Autodesk Inventor part; units mm, degrees
ref_plane "YZ Plane" through (0, 0, 0) normal (1, 0, 0) x (0, 1, 0)
ref_plane "XZ Plane" through (0, 0, 0) normal (0, 1, 0) x (-1, 0, 0)
ref_plane "XY Plane" through (0, 0, 0) normal (0, 0, 1) x (1, 0, 0)
sketch "Sketch1" plane through (0, 0, 0) normal (0, 0, 1) x (1, 0, 0)
  line L0 (0, 0) -> (31.75, 0) construction
  line L1 (31.75, 0) -> (44.45, 0)
  line L2 (44.45, 0) -> (44.45, -19.05)
  line L3 (44.45, -19.05) -> (38.1, -30.0485)
  line L4 (38.1, -30.0485) -> (38.1, -42.7485)
  line L5 (38.1, -42.7485) -> (44.45, -53.747)
  line L6 (44.45, -53.747) -> (44.45, -88.9)
  line L7 (44.45, -88.9) -> (31.75, -88.9)
  line L8 (31.75, -88.9) -> (31.75, 0)
  line L9 (0, 0) -> (0, -152.4)
  dimension "d0" = 31.75
  dimension "d1" = 12.7
  dimension "d2" = 6.35
  dimension "d3" = 150
  dimension "d4" = 19.05
  dimension "d5" = 88.9
  dimension "d6" = 150
  dimension "d7" = 12.7
  dimension "d9" = 152.4
revolve "Revolution1" add sketch "Sketch1" angle 270 about axis through (0, 0, 0) along (0, -1, 0)
fillet "Fillet1" radius 12.7 2 edges at (-31.4309, -19.05, 31.4309) (-31.4309, -53.747, 31.4309)
fillet "Fillet1" radius 6.35 2 edges at (-26.9408, -42.7485, 26.9408) (-26.9408, -30.0485, 26.9408)
equation "\"d6\" = d3"
properties part number "Foam Weight Shifter Pad 1"
Verification items for the finished model (mm, model axes). A direction names the side the tool comes from. Give positions to 0.01 mm unless a question says otherwise; leave off trailing zeros. Order: outer loops, then holes, each group sorted by start corner. A loop starts at its lowest first (then second) coordinate and runs counter-clockwise, first axis right, second up. Notation, with made-up numbers: M -37.5,6 L -22.5,6 A23 ccw -22.5,25 Z; hole C -9,-39 d1. An arc over 180 degrees is marked long. Return JSON: item names as keys, results as strings. Group by question number.
1) Access from +Z, -Z, +X, -X, +Y, -Y to the whole of each face (thin tool, end or side, straight path). Record for faces 1 (the face through (-26.78, -44.63, 28.61)), 2 (the face through (0, -44, -38)), 3 (the face through (-30.38, -7.93, 32.45)).
2) Section check A-A on y = -81.5. Record the cut outline in (x, z).
3) Go/stop test with flat-tipped pins: pin 1 Ø1 at (y, z) = (-37.5, 12.5) entering from +X; pin 2 Ø6.5 at (x, y) = (41, -46) entering from -Z; pin 3 Ø10 at (y, z) = (-65, -36) entering from +X. Record where each tip stops, or that it passes through.
4) Scan lines: line 1 (Y direction, x = -14.5, z = -38); line 2 (Z direction, x = -21.5, y = -67.5); line 3 (X direction, y = -11, z = 19). Record each from-to range of solid material in increasing order.
5) Mould release check, pull along Y, two halves, no side actions. Record for faces 4 (the face through (-26.04, -36.46, 27.81)), 5 (the face through (-23, -88.9, 23)), 6 (the face through (-23.179, -43.828, 21.698)): pulls with the +Y half, pulls with the -Y half, needs draft (parallel to the pull), parting line crosses it, or undercut.
Answer block:
{
 "1": {"face 1": "none", "face 2": "-Z, +X, +Y, -Y", "face 3": "+Y, -Y"},
 "2": {"outline": "M 0,-44.45 L 0,-31.75 A31.75 cw long 31.75,0 L 44.45,0 A44.45 ccw long Z"},
 "3": {"pin 1": "stops at x = 36.16", "pin 2": "stops at z = 0", "pin 3": "stops at x = 0"},
 "4": {"line 1": "y = -88.9 to -47.2, -25.59 to 0", "line 2": "z = -38.9 to -23.36, 23.36 to 38.9", "line 3": "x = -40.18 to -25.44, 25.44 to 40.18"},
 "5": {"face 4": "undercut", "face 5": "pulls with the -Y half", "face 6": "needs draft"}
}
